Source: CAD feature listing. Evaluate the final solid. Frame: model axes, mm. A direction names the side the tool comes from. Give positions to 0.01 mm unless a question says otherwise; leave off trailing zeros. Write each loop counter-clockwise with the first axis right and the second up, starting at its lowest first coordinate (ties: lowest second). Pieces come first, ordered by that corner, then holes. Notation, with made-up numbers: (70.25, -19) - (123.25, -19) arc R22 ccw to (123.25, -5) - close; hole circle Ø9 at (-2.5, 61.5). An arc over 180 degrees is marked (long way). Answer as a JSON object with one key per item and string values. Group by question number.
from build123d import *

# Parameters (mm, degrees)
BOSS_EXTRUDE1_DEPTH     = 50
CUT_EXTRUDE1_DEPTH      = 92.586319753
CUT_EXTRUDE1_DEPTH_BACK = 92.586319753
CUT_EXTRUDE2_DEPTH      = 98.796895786
CUT_EXTRUDE2_DEPTH_BACK = 15
SKETCH3_R               = 4


with BuildPart() as part:
    # Sketch1 → Boss-Extrude1 (new, symmetric)
    with BuildSketch(Plane.XY):
        with BuildLine():
            Line((-11.48444402, 0), (-12.5, 0))
            Line((-12.5, 0), (-12.5, 8))
            Line((-12.5, 8), (12.5, 8))
            Line((12.5, 8), (12.5, 0))
            Line((12.5, 0), (9.300622615, 0))
            ThreePointArc((9.300622615, 0), (7.579893306, -0.542543867), (6.481544752, -1.97393957))
            Line((6.481544752, -1.97393957), (-18.1, -69.511178712))
            Line((-18.1, -69.511178712), (-32.5, -69.511178712))
            Line((-32.5, -69.511178712), (-8.665366158, -4.02606043))
            ThreePointArc((-8.665366158, -4.02606043), (-9.026987887, -1.279270691), (-11.48444402, 0))
        make_face()
    extrude(amount=BOSS_EXTRUDE1_DEPTH, both=True)

    # Sketch2 → Cut-Extrude1 (cut, two sides: drawn at the far end of the back side and taken through both)
    with BuildSketch(Plane(origin=(0, 0, 0), x_dir=(0, 0, -1), z_dir=(1, 0, 0)).offset(-CUT_EXTRUDE1_DEPTH_BACK)):
        with BuildLine():
            Line((40, -7), (-40, -7))
            Line((-40, -7), (-40, -49.511178712))
            ThreePointArc((-40, -49.511178712), (-37.071067812, -56.582246524), (-30, -59.511178712))
            Line((-30, -59.511178712), (30, -59.511178712))
            ThreePointArc((30, -59.511178712), (37.071067812, -56.582246524), (40, -49.511178712))
            Line((40, -49.511178712), (40, -7))
        make_face()
        with BuildLine():
            Line((-50, -49.511178712), (-50, -69.511178712))
            Line((-50, -69.511178712), (-30, -69.511178712))
            ThreePointArc((-30, -69.511178712), (-44.142135624, -63.653314336), (-50, -49.511178712))
        make_face()
        with BuildLine():
            Line((50, -49.511178712), (50, -69.511178712))
            Line((50, -69.511178712), (30, -69.511178712))
            ThreePointArc((30, -69.511178712), (44.142135624, -63.653314336), (50, -49.511178712))
        make_face()
    extrude(amount=CUT_EXTRUDE1_DEPTH + CUT_EXTRUDE1_DEPTH_BACK, mode=Mode.SUBTRACT)

    # Sketch3 → Cut-Extrude2 (cut, two sides: drawn at the far end of the back side and taken through both)
    with BuildSketch(Plane(origin=(0, 8, 0), x_dir=(1, 0, 0), z_dir=(0, 1, 0)).offset(-CUT_EXTRUDE2_DEPTH_BACK)):
        with Locations(Location((0, -25, 0), (0, 0, 270))):
            Circle(SKETCH3_R)
        with Locations(Location((0, 25, 0), (0, 0, 270))):
            Circle(SKETCH3_R)
    extrude(amount=CUT_EXTRUDE2_DEPTH + CUT_EXTRUDE2_DEPTH_BACK, mode=Mode.SUBTRACT)


solid = part.part
Q1. Section D-D on x = -20. Return the cut outline in (y, z), then the cut area to 3 significant figures.
Q2. Section C-C on x = 0. Return the cut outline in (y, z).
Q3. Section B-B on z = 18.5. Return the cut outline in (x, y), then the cut area to 3 significant figures.
Q4. Draft query along Y for faces 1 (the cylindrical face through (-2.4, 0.4, 21.8)), 2 (the cylindrical face through (-9.004, -1.312, 0.7)), 3 (the flat face through (-25, -69.511, 0)). Return one class per face: released by +Y, released by -Y, zero draft, split by the parting line, or undercut.
Q5. First-contact query: pin 1 Ø7 at (x, z) = (-20, 2) entering from +Y; pin 2 Ø4.5 at (x, z) = (-4, -19) entering from -Y; pin 3 Ø6.5 at (y, z) = (5.5, 3.5) entering from -X. Flat tips, straight axial feed; report the tip coordinate or a pass-through.
Q6. Reachability of faces 4 (the flat face through (-29.466, -61.175, 3.937)), 5 (the flat face through (-3, -7, -1)), 6 (the flat face through (-10, -29, -40)) from +Z, -Z, +X, -X, +Y, -Y: full face, straight path, thin tool, end or side. Return the list, or none.
Q7. Section A-A on z = -25. Return the cut outline in (x, y).
Q8. Ray query, probe 1 along Z at (x, y) = (0, 2.5); probe 2 along X at (y, z) = (4.75, -25); probe 3 along Z at (x, y) = (1, -10). Return the intervals inside material, ascending. Write a range as [from, to].
Taken from the geometry:
{
 "1": {"outline": "(-69.51, -30) arc R20 ccw to (-49.51, -50) - (-35.17, -50) - (-35.17, -40) - (-49.51, -40) arc R10 cw to (-59.51, -30) - (-59.51, 30) arc R10 cw to (-49.51, 40) - (-35.17, 40) - (-35.17, 50) - (-49.51, 50) arc R20 ccw to (-69.51, 30) - close", "area": "1,360 mm²"},
 "2": {"outline": "(-19.78, -50) - (8, -50) - (8, -29) - (-7, -29) - (-7, -40) - (-19.78, -40) - close; (-19.78, 40) - (-7, 40) - (-7, 29) - (8, 29) - (8, 50) - (-19.78, 50) - close; (-7, -21) - (8, -21) - (8, 21) - (-7, 21) - close"},
 "3": {"outline": "(-32.5, -69.51) - (-18.1, -69.51) - (-14.46, -59.51) - (-28.86, -59.51) - close; (-12.5, 0) - (-11.48, 0) arc R3 cw to (-8.67, -4.03) - (-9.75, -7) - (4.65, -7) - (6.48, -1.97) arc R3 cw to (9.3, 0) - (12.5, 0) - (12.5, 8) - (-12.5, 8) - close", "area": "450 mm²"},
 "4": {"face 1": "zero draft", "face 2": "undercut", "face 3": "released by -Y"},
 "5": {"pin 1": "stops at y = -59.51", "pin 2": "stops at y = -7", "pin 3": "stops at x = -12.5"},
 "6": {"face 4": "+Z, -Z, -X", "face 5": "+X, -X, -Y", "face 6": "+X, -X"},
 "7": {"outline": "(-32.5, -69.51) - (-18.1, -69.51) - (-14.46, -59.51) - (-28.86, -59.51) - close; (-12.5, 0) - (-11.48, 0) arc R3 cw to (-8.67, -4.03) - (-9.75, -7) - (-4, -7) - (-4, 8) - (-12.5, 8) - close; (4, -7) - (4.65, -7) - (6.48, -1.97) arc R3 cw to (9.3, 0) - (12.5, 0) - (12.5, 8) - (4, 8) - close"},
 "8": {"probe 1": "z = [-50, -29], [-21, 21], [29, 50]", "probe 2": "x = [-12.5, -4], [4, 12.5]", "probe 3": "z = [-50, -40], [40, 50]"}
}
